from build123d import *

# Parameters (mm, degrees)
SKETCH_W        = 20
SKETCH_H        = 22
PAD_DEPTH       = 1
SKETCH001_W     = 8.5
SKETCH001_H     = 6.5
POCKET_DEPTH    = 0.5
SKETCH002_W     = 2.142857
SKETCH002_H     = 5
SKETCH002_W_2   = 2.142858
POCKET001_DEPTH = 5


with BuildPart() as part:
    # Sketch → Pad (new body)
    with BuildSketch(Plane.XZ):
        Rectangle(SKETCH_W, SKETCH_H)
    extrude(amount=PAD_DEPTH)

    # Sketch001 (on Face6 of Pad) → Pocket (cut)
    with BuildSketch(Plane.XZ.offset(1)):
        with Locations((-4.75, 0.75)):
            Rectangle(SKETCH001_W, SKETCH001_H)
        with Locations((-4.75, -6.75)):
            Rectangle(SKETCH001_W, SKETCH001_H)
        with Locations((4.75, 0.75)):
            Rectangle(SKETCH001_W, SKETCH001_H)
        with Locations((4.75, -6.75)):
            Rectangle(SKETCH001_W, SKETCH001_H)
    extrude(amount=-POCKET_DEPTH, mode=Mode.SUBTRACT)

    # Sketch002 (on Face5 of Pocket) → Pocket001 (cut)
    with BuildSketch(Plane.XZ.offset(1)):
        with Locations((-7.928572, 7.5)):
            Rectangle(SKETCH002_W, SKETCH002_H)
        with Locations((-5.285714, 7.5)):
            Rectangle(SKETCH002_W, SKETCH002_H)
        with Locations((-2.642857, 7.5)):
            Rectangle(SKETCH002_W, SKETCH002_H)
        with Locations((0, 7.5)):
            Rectangle(SKETCH002_W_2, SKETCH002_H)
        with Locations((2.642857, 7.5)):
            Rectangle(SKETCH002_W, SKETCH002_H)
        with Locations((5.285714, 7.5)):
            Rectangle(SKETCH002_W, SKETCH002_H)
        with Locations((7.928572, 7.5)):
            Rectangle(SKETCH002_W, SKETCH002_H)
    extrude(amount=-POCKET001_DEPTH, mode=Mode.SUBTRACT)


solid = part.part
Here's how the part is built. I have some questions about the finished solid (model axes, mm). A direction names the side the tool comes from. Give positions to 0.01 mm unless a question says otherwise; leave off trailing zeros. Loops run counter-clockwise (first coordinate to the right, second up) from the corner with the lowest first, then second, coordinate; pieces in that order, holes last. Notation, with made-up numbers: (-24, 6) -> (-15, 6) arc R12 ccw to (-15, 15) -> close; hole circle Ø7 at (-13.5, 87). An arc over 180 degrees is marked (long way). Answer as a JSON object with one key per item and string values. Group by question number.
Item 1: Imagine slicing it at D-D on z = -8. Write out the boundary of the cut face in (x, y).
Item 2: Imagine slicing it at B-B on y = -0.3. Give the number of separate pieces and of enclosed holes in the cut face, then the cut area to 3 significant figures.
Item 3: I need wall thicknesses on L1, parallel to Z at x = -7.5, y = -0.7; L2, parallel to X at y = -0.75, z = -8.75; L3, parallel to Z at x = -3, y = -0.15. Which ranges of each line are inside material? Lowest first, please.
Item 4: Thinking about a two-plate mould opening in Z: for faces 1 (the flat face through (5, -0.5, 1)), 2 (the flat face through (-0.1, -0.5, -11)), which applies, pulls with the +Z half, pulls with the -Z half, needs draft (parallel to the pull), parting line crosses it, or undercut?
Item 5: On a 3-axis mill with a long thin cutter (end or side, diameter ignored), from which of +Z, -Z, +X, -X, +Y, -Y can I reach the whole of each face in a straight line? I mean faces 3 (the flat face through (-5.3, -0.5, 10)), 4 (the flat face through (5, -0.5, -7)). Say none if no direction works.
Item 6: Imagine slicing it at A-A on x = 2. Write out the boundary of the cut face in (y, z).
Item 7: Will this pin go through, and if not, where does the flat tip stop? pin 1 (3 mm diameter, centred on x = 6.5, z = 2, fed in from -Y).
Answer list:
{
 "1": {"outline": "(-10, -1) -> (-9, -1) -> (-9, -0.5) -> (-0.5, -0.5) -> (-0.5, -1) -> (0.5, -1) -> (0.5, -0.5) -> (9, -0.5) -> (9, -1) -> (10, -1) -> (10, 0) -> (-10, 0) -> close"},
 "2": {"separate pieces": "1", "enclosed holes": "7", "area": "365 mm2"},
 "3": {"L1": "z = -11 to -10, -3.5 to -2.5, 4 to 5, 10 to 11", "L2": "x = -10 to -9, -0.5 to 0.5, 9 to 10", "L3": "z = -11 to 5, 10 to 11"},
 "4": {"face 1": "undercut", "face 2": "pulls with the -Z half"},
 "5": {"face 3": "+Y, -Y", "face 4": "-Y"},
 "6": {"outline": "(-1, -11) -> (0, -11) -> (0, 5) -> (-1, 5) -> (-1, 4) -> (-0.5, 4) -> (-0.5, -2.5) -> (-1, -2.5) -> (-1, -3.5) -> (-0.5, -3.5) -> (-0.5, -10) -> (-1, -10) -> close; (-1, 10) -> (0, 10) -> (0, 11) -> (-1, 11) -> close"},
 "7": {"pin 1": "stops at y = -0.5"}
}
